Check sheet for the modelled part. Datum: model origin and axes. Units: mm. Give positions to 0.01 mm unless a question says otherwise; leave off trailing zeros. Order: outer loops, then holes, each group sorted by start corner. A loop starts at its lowest first (then second) coordinate and runs counter-clockwise, first axis right, second up.
from build123d import *

# Parameters (mm, degrees)
CUBO_START          = 20.5
SK_CUBO_R           = 17
CUBO_DEPTH          = 14
PASANTES_M2_5_START = 20.5
SK_PASANTES_M2_5_R  = 1.45
PASANTES_M2_5_DEPTH = 14
CENTRO_START        = 20.5
SK_CENTRO_R         = 3
CENTRO_DEPTH        = 14


with BuildPart() as part:
    # Sk_Cubo → Cubo (new body)
    with BuildSketch(Plane(origin=(0, 0, 0), x_dir=(1, 0, 0), z_dir=(0, 1, 0)).offset(CUBO_START)):
        with Locations(Location((0, -490, 0), (0, 0, 270))):
            Circle(SK_CUBO_R)
    extrude(amount=CUBO_DEPTH)

    # Sk_Pasantes_M2-5 → Pasantes_M2-5 (cut)
    with BuildSketch(Plane(origin=(0, 0, 0), x_dir=(1, 0, 0), z_dir=(0, 1, 0)).offset(PASANTES_M2_5_START)):
        with Locations(Location((12.390194253, -491.653204878, 0), (0, 0, 270))):
            Circle(SK_PASANTES_M2_5_R)
        with Locations(Location((4.763379704, -501.55682542, 0), (0, 0, 270))):
            Circle(SK_PASANTES_M2_5_R)
        with Locations(Location((-7.626814549, -499.903620542, 0), (0, 0, 270))):
            Circle(SK_PASANTES_M2_5_R)
        with Locations(Location((-12.390194253, -488.346795122, 0), (0, 0, 270))):
            Circle(SK_PASANTES_M2_5_R)
        with Locations(Location((-4.763379704, -478.44317458, 0), (0, 0, 270))):
            Circle(SK_PASANTES_M2_5_R)
        with Locations(Location((7.626814549, -480.096379458, 0), (0, 0, 270))):
            Circle(SK_PASANTES_M2_5_R)
    extrude(amount=PASANTES_M2_5_DEPTH, mode=Mode.SUBTRACT)

    # Sk_Centro → Centro (cut)
    with BuildSketch(Plane(origin=(0, 0, 0), x_dir=(1, 0, 0), z_dir=(0, 1, 0)).offset(CENTRO_START)):
        with Locations(Location((0, -490, 0), (0, 0, 270))):
            Circle(SK_CENTRO_R)
    extrude(amount=CENTRO_DEPTH, mode=Mode.SUBTRACT)


solid = part.part
1) Draft check along X on faces 1 (the face through (0.747, 27.402, 473.016)), 2 (the face through (-4, 34.5, 490)), 3 (the face through (7.691, 27.402, 478.648)). Enter one of: +X half, -X half, draft (parallel to the pull), parting line (faces both ways), or undercut.
Recorded:
face 1: parting line
face 2: draft
face 3: undercut
2) Section check C-C, the plane z = 480.5. Record the cut outline in (x, y), then the cut area to 3 significant figures.
Recorded:
outline: (-14.1, 20.5) - (6.23, 20.5) - (6.23, 34.5) - (-14.1, 34.5) - close; (9.02, 20.5) - (14.1, 20.5) - (14.1, 34.5) - (9.02, 34.5) - close
area: 356 mm2
3) Depth check by flat-ended pin: pin 1 Ø4 at (y, z) = (29, 482) entering from -X; pin 2 Ø6 at (x, y) = (7.5, 28.5) entering from +Z; pin 3 Ø6 at (x, y) = (-12, 23.5) entering from +Z. Enter the tip coordinate at first touch or a pass-through.
Recorded:
pin 1: stops at x = -15.91
pin 2: stops at z = 506.39
pin 3: stops at z = 504.42
4) Section check D-D, the plane y = 26.25. Record the cut outline in (x, z).
Recorded:
outline: circle Ø34 at (0, 490); hole circle Ø2.9 at (-12.39, 488.35); hole circle Ø2.9 at (-7.63, 499.9); hole circle Ø2.9 at (-4.76, 478.44); hole circle Ø6 at (0, 490); hole circle Ø2.9 at (4.76, 501.56); hole circle Ø2.9 at (7.63, 480.1); hole circle Ø2.9 at (12.39, 491.65)
5) Section check B-B, the plane z = 491. Record the cut outline in (x, y).
Recorded:
outline: (-16.97, 20.5) - (-2.83, 20.5) - (-2.83, 34.5) - (-16.97, 34.5) - close; (2.83, 20.5) - (11.1, 20.5) - (11.1, 34.5) - (2.83, 34.5) - close; (13.68, 20.5) - (16.97, 20.5) - (16.97, 34.5) - (13.68, 34.5) - close
6) Material ranges on L1, parallel to X at y = 30.5, z = 488.5; L2, parallel to X at y = 27, z = 490; L3, parallel to X at y = 22.25, z = 488, recorded low to high.
Recorded:
L1: x = -16.93 to -13.83, -10.95 to -2.6, 2.6 to 16.93
L2: x = -17 to -3, 3 to 17
L3: x = -16.88 to -13.8, -10.98 to -2.24, 2.24 to 16.88
7) Section check A-A, the plane x = 0. Record the cut outline in (y, z), then the cut area to 3 significant figures.
Recorded:
outline: (20.5, 473) - (34.5, 473) - (34.5, 487) - (20.5, 487) - close; (20.5, 493) - (34.5, 493) - (34.5, 507) - (20.5, 507) - close
area: 392 mm2
